from build123d import *

# Parameters (mm, degrees)
SKETCH049_R      = 2
EXTRUDE050_DEPTH = 15
SKETCH044_W      = 35
SKETCH044_H      = 14
EXTRUDE043_DEPTH = 15
SKETCH040_R      = 1.5
SKETCH040_W      = 20
SKETCH040_H      = 4
EXTRUDE039_DEPTH = 2


with BuildPart() as weapon_cover_screw_holes001:
    # Sketch049 (on Face6 of Cut025) → Extrude050 (new body, symmetric)
    with BuildSketch(Plane.XY.offset(39.2)):
        with Locations((-29.074951, -82.714325)):
            Circle(SKETCH049_R)
        with Locations((13.75458, -82.714325)):
            Circle(SKETCH049_R)
        with Locations((-29.074951, -19.516283)):
            Circle(SKETCH049_R)
        with Locations((13.75458, -19.516283)):
            Circle(SKETCH049_R)
    extrude(amount=EXTRUDE050_DEPTH, both=True)


with BuildPart() as servo_lid_gap:
    # Sketch044 (on Face8 of Cut013) → Extrude043 (new body, symmetric)
    with BuildSketch(Plane.XY.offset(38)):
        with Locations((0, -51.440889)):
            Rectangle(SKETCH044_W, SKETCH044_H)
    extrude(amount=EXTRUDE043_DEPTH, both=True)


with BuildPart() as lid:
    # Sketch040 (on Face4 of Cut018) → Extrude039 (new body)
    with BuildSketch(Plane.XY.offset(35)):
        with BuildLine():
            Line((-60, 35.090242), (60, 35.090242))
            Line((60, 35.090242), (60, -34.909758))
            Line((60, -34.909758), (95, -34.909758))
            Line((95, -34.909758), (95, -89.909758))
            ThreePointArc((-95, -89.909758), (0, -121.776758), (95, -89.909758))
            Line((-95, -34.909758), (-95, -89.909758))
            Line((-60, -34.909758), (-95, -34.909758))
            Line((-60, 35.090242), (-60, -34.909758))
        make_face()
        with Locations((70.898361, -39.7159)):
            Circle(SKETCH040_R, mode=Mode.SUBTRACT)
        with Locations((37.389542, 29.290899)):
            Circle(SKETCH040_R, mode=Mode.SUBTRACT)
        with Locations((-37.606323, 29.30405)):
            Circle(SKETCH040_R, mode=Mode.SUBTRACT)
        with Locations((-67.618576, -39.684311)):
            Circle(SKETCH040_R, mode=Mode.SUBTRACT)
        with Locations((0.80288, -92.081482)):
            Rectangle(SKETCH040_W, SKETCH040_H, mode=Mode.SUBTRACT)
    extrude(amount=EXTRUDE039_DEPTH)

    # Cut022: cut Servo Lid Gap
    add(servo_lid_gap.part, mode=Mode.SUBTRACT)

    # Cut027: cut Weapon Cover Screw Holes001
    add(weapon_cover_screw_holes001.part, mode=Mode.SUBTRACT)


solid = lid.part
Verification items for the finished model (mm, model axes). Give positions to 0.01 mm unless a question says otherwise; leave off trailing zeros. Write each loop counter-clockwise with the first axis right and the second up, starting at its lowest first coordinate (ties: lowest second). Pieces come first, ordered by that corner, then holes. Notation, with made-up numbers: M 43,61.25 L 65,61.25 A24 cw 65,82.25 Z; hole C 49.5,72 d9. An arc over 180 degrees is marked long. Put each result on its own line as item: value. Start each with the question number.
1. Section check D-D (x = -62). Record the cut outline in (y, z).
2. Draft check along Y on faces 1 (the face through (-29.34, -80.73, 36.01)), 2 (the face through (-1.43, -121.77, 35.99)), 3 (the face through (1, -42, 35)). Enter one of: +Y half, -Y half, draft (parallel to the pull), parting line (faces both ways), or undercut.
3. Section check B-B (z = 36). Give the number of separate pieces and of enclosed holes in the cut face, and give its area (3 significant figures).
4. Scan lines: line 1 along Y through (x, z) = (1, 35.1); line 2 along X through (y, z) = (12, 35.35); line 3 along Y through (x, z) = (5.5, 35.8). Record each from-to range of solid material in increasing order. Write a range as [from, to].
5. Section check C-C (y = -9). Record the cut outline in (x, z), and give its area (3 significant figures).
6. Go/stop test with flat-tipped pins: pin 1 Ø1 at (x, z) = (-84.5, 35.5) entering from +Y; pin 2 Ø1 at (y, z) = (1, 36) entering from +X. Record where each tip stops, or that it passes through.
7. Section check A-A (x = -2). Record the cut outline in (y, z), and give its area (3 significant figures).
Answer list:
1. outline: M -109.06,35 L -34.91,35 L -34.91,37 L -109.06,37 Z
2. face 1: undercut
2. face 2: -Y half
2. face 3: draft
3. separate pieces: 1
3. enclosed holes: 10
3. area: 22,300 mm2
4. line 1: [-121.77, -94.08], [-90.08, -58.44], [-44.44, 35.09]
4. line 2: [-60, 60]
4. line 3: [-121.68, -94.08], [-90.08, -58.44], [-44.44, 35.09]
5. outline: M -60,35 L 60,35 L 60,37 L -60,37 Z
5. area: 240 mm2
6. pin 1: y = -34.91
6. pin 2: x = 60
7. outline: M -121.76,35 L -94.08,35 L -94.08,37 L -121.76,37 Z; M -90.08,35 L -58.44,35 L -58.44,37 L -90.08,37 Z; M -44.44,35 L 35.09,35 L 35.09,37 L -44.44,37 Z
7. area: 278 mm2
